```python
from build123d import *

# Parameters (mm, degrees)
SKETCH1_R           = 2.76225
BOSS_EXTRUDE1_DEPTH = 3.3655
SKETCH2_W           = 13.1318
SKETCH2_H           = 3.2766
BOSS_EXTRUDE2_DEPTH = 1.0541
FILLET1_R           = 1.651
SKETCH3_R           = 0.635
CUT_EXTRUDE1_DEPTH  = 3.3655
SKETCH4_R           = 1.49225
CUT_EXTRUDE2_DEPTH  = 2.54
SKETCH5_R           = 0.45085
CUT_EXTRUDE3_DEPTH  = 14.834720946


with BuildPart() as part:
    # Sketch1 → Boss-Extrude1 (new body)
    with BuildSketch(Plane.XY):
        Circle(SKETCH1_R)
    extrude(amount=BOSS_EXTRUDE1_DEPTH)

    # Sketch2 → Boss-Extrude2 (add)
    with BuildSketch(Plane.XY.offset(3.3655)):
        with Locations((6.5659, 0)):
            Rectangle(SKETCH2_W, SKETCH2_H)
    extrude(amount=-BOSS_EXTRUDE2_DEPTH)

    # Fillet1
    # the kernel refuses this fillet: 1.651 mm, written as the material it takes off along each edge
    with BuildSketch(Plane(origin=(13.1318, -1.6383, 7.493), x_dir=(-1, 0, 0), z_dir=(0, 0, -1))) as fillet1_piece_1:
        with BuildLine():
            CenterArc((FILLET1_R, FILLET1_R), FILLET1_R, 180, 90)
            Line((0, FILLET1_R), (0, 0))
            Line((0, 0), (FILLET1_R, 0))
        make_face()
    extrude(amount=9.3091, mode=Mode.SUBTRACT)
    with BuildSketch(Plane(origin=(13.1318, 1.6383, 7.493), x_dir=(-1, 0, 0), z_dir=(0, 0, -1))) as fillet1_piece_2:
        with BuildLine():
            CenterArc((FILLET1_R, -FILLET1_R), FILLET1_R, 90, 90)
            Line((0, -FILLET1_R), (0, 0))
            Line((0, 0), (FILLET1_R, 0))
        make_face()
    extrude(amount=9.3091, mode=Mode.SUBTRACT)

    # Sketch3 → Cut-Extrude1 (cut)
    with BuildSketch(Plane.XY.offset(3.3655)):
        Circle(SKETCH3_R)
    extrude(amount=-CUT_EXTRUDE1_DEPTH, mode=Mode.SUBTRACT)

    # Sketch4 → Cut-Extrude2 (cut)
    with BuildSketch(Plane(origin=(0, 0, 0), x_dir=(-1, 0, 0), z_dir=(0, 0, -1))):
        Circle(SKETCH4_R)
    extrude(amount=-CUT_EXTRUDE2_DEPTH, mode=Mode.SUBTRACT)

    # Sketch5 → Cut-Extrude3 (cut, through all)
    with BuildSketch(Plane.XY.offset(3.3655)):
        with Locations((6.858, 0)):
            Circle(SKETCH5_R)
        with Locations((9.398, 0)):
            Circle(SKETCH5_R)
        with Locations((11.938, 0)):
            Circle(SKETCH5_R)
    extrude(amount=-CUT_EXTRUDE3_DEPTH, mode=Mode.SUBTRACT)


solid = part.part
```
Work out the finished part from the listing and answer in its coordinate system (mm). A direction names the side the tool comes from. Round coordinates to 2 decimals unless told otherwise and drop trailing zeros. Loops run counter-clockwise (first coordinate to the right, second up) from the corner with the lowest first, then second, coordinate; pieces in that order, holes last. Notation, with made-up numbers: (21, 28) -> (32, 28) arc R18 cw to (32, 36) -> close; hole circle Ø10 at (20.25, 63). An arc over 180 degrees is marked (long way). Write each question's results on one line, items separated by ' | '. Start each with the question number.
1. Given pin 1 Ø3 at (x, y) = (9, 0) entering from -Z; pin 2 Ø0.8 at (x, z) = (7.5, 2.5) entering from +Y; pin 3 Ø1.2 at (x, z) = (7, 3) entering from -Y, each flat-ended and moving along its own axis, determine where each tip first touches the part or whether it passes through.
2. Section C-C (x = 12.25) is taken. Determine the outline of the cut face in (y, z).
3. Find the intervals of material crossed by probe 1 along Y at (x, z) = (0, 0.85); probe 2 along Y at (x, z) = (0, 3) (3 decimals); probe 3 along X at (y, z) = (-0.2, 3.2) (3 decimals), in increasing order. Write a range as from..to.
4. For a pull along Y with two mould halves and no side action, classify faces 1 (the face through (1.2, -1.2, 0)), 2 (the face through (12.7, -1.1, 2.8)), 3 (the face through (-1, 0, 2.54)) as +Y half, -Y half, draft (parallel to the pull), parting line (faces both ways), or undercut.
5. Section D-D (z = 0.3) is taken. Determine the outline of the cut face in (x, y), plus the area to 3 significant figures.
6. Section A-A (z = 2.7) is taken. Determine the outline of the cut face in (x, y) (1 decimal).
7. Section B-B (x = 0) is taken. Determine the outline of the cut face in (y, z) (1 decimal), plus the area to 3 significant figures.
8. A tool of negligible diameter and unlimited length cuts with its end or side. For faces 4 (the face through (7, 1.638, 3)), 5 (the face through (7, -1.638, 3)), 6 (the face through (5, 0, 3.366)), 7 (the face through (11.488, 0.02, 2.846)), 8 (the face through (0.323, -1.457, 1.252)), from which of +Z, -Z, +X, -X, +Y, -Y can it reach the whole face along a straight path? Write none if from no direction.
Evaluation:
1) pin 1: stops at z = 2.31 | pin 2: stops at y = 1.64 | pin 3: stops at y = -1.64
2) outline: (-1.45, 2.31) -> (-0.33, 2.31) -> (-0.33, 3.37) -> (-1.45, 3.37) -> close; (0.33, 2.31) -> (1.45, 2.31) -> (1.45, 3.37) -> (0.33, 3.37) -> close
3) probe 1: y = -2.76..-1.49, 1.49..2.76 | probe 2: y = -2.762..-0.635, 0.635..2.762 | probe 3: x = -2.755..-0.603, 0.603..6.454, 7.262..8.994, 9.802..11.534, 12.342..13.118
4) face 1: draft | face 2: -Y half | face 3: undercut
5) outline: circle Ø5.52 at (0, 0); hole circle Ø2.98 at (0, 0) | area: 17.0 mm2
6) outline: (2.2, -1.6) -> (11.5, -1.6) arc R1.7 ccw to (13.1, 0) arc R1.7 ccw to (11.5, 1.6) -> (2.2, 1.6) arc R2.8 ccw (long way) to start; hole circle Ø1.3 at (0, 0); hole circle Ø0.9 at (6.9, 0); hole circle Ø0.9 at (9.4, 0); hole circle Ø0.9 at (11.9, 0)
7) outline: (-2.8, 0) -> (-1.5, 0) -> (-1.5, 2.5) -> (-0.6, 2.5) -> (-0.6, 3.4) -> (-2.8, 3.4) -> close; (0.6, 2.5) -> (1.5, 2.5) -> (1.5, 0) -> (2.8, 0) -> (2.8, 3.4) -> (0.6, 3.4) -> close | area: 9.96 mm2
8) face 4: +Z, -Z, +X, +Y | face 5: +Z, -Z, +X, -Y | face 6: +Z, +X, -X, +Y, -Y | face 7: +Z, -Z | face 8: -Z
